Can you work these out from the model? Positions are in its coordinate system, mm. A direction names the side the tool comes from. Give positions to 0.01 mm unless a question says otherwise; leave off trailing zeros. Loops run counter-clockwise (first coordinate to the right, second up) from the corner with the lowest first, then second, coordinate; pieces in that order, holes last. Notation, with made-up numbers: M -39,-36.75 L 0,-36.75 A26 ccw 0,-8.75 Z; hole C 4,6.5 d2. An arc over 180 degrees is marked long. One line per item, written item: value. Start each with the question number.
from build123d import *

# Parameters (mm, degrees)
SKETCH2_R          = 27.5
CUT_EXTRUDE1_DEPTH = 4
CUT_EXTRUDE2_DEPTH = 28


with BuildPart() as part:
    # Sketch1 → Revolve1 (revolve)
    with BuildSketch(Plane(origin=(0, 0, 0), x_dir=(0, 0, -1), z_dir=(1, 0, 0))):
        with BuildLine():
            Line((0, 0), (43, 0))
            Line((43, 0), (43, -5))
            Line((43, -5), (44, -5))
            ThreePointArc((44, -5), (44.707106781, -4.707106781), (45, -4))
            Line((45, -4), (45, -1))
            ThreePointArc((45, -1), (44.121320344, 1.121320344), (42, 2))
            Line((42, 2), (41, 2))
            ThreePointArc((41, 2), (38.878679656, 2.878679656), (38, 5))
            Line((38, 5), (38, 9))
            ThreePointArc((38, 9), (37.121320344, 11.121320344), (35, 12))
            Line((35, 12), (0, 12))
            Line((0, 12), (0, 0))
        make_face()
    revolve(axis=Axis((0, 12, 0), (0, -1, 0)))

    # Sketch2 → Cut-Extrude1 (cut)
    with BuildSketch(Plane(origin=(0, 12, 0), x_dir=(1, 0, 0), z_dir=(0, 1, 0))):
        with Locations((0, -2.368290616)):
            Circle(SKETCH2_R)
    extrude(amount=-CUT_EXTRUDE1_DEPTH, mode=Mode.SUBTRACT)

    # Sketch3 → Cut-Extrude2 (cut)
    with BuildSketch(Plane(origin=(0, 12, 0), x_dir=(1, 0, 0), z_dir=(0, 1, 0))):
        with BuildLine():
            Line((-6.5, 32.565854692), (6.5, 32.565854692))
            ThreePointArc((6.5, 32.565854692), (9, 30.065854692), (6.5, 27.565854692))
            Line((6.5, 27.565854692), (-6.5, 27.565854692))
            ThreePointArc((-6.5, 27.565854692), (-9, 30.065854692), (-6.5, 32.565854692))
        make_face()
    extrude(amount=-CUT_EXTRUDE2_DEPTH, mode=Mode.SUBTRACT)


solid = part.part
Q1. If we section it at D-D, the plane y = 3.75: Write out the boundary of the cut face in (x, z), plus the area to 3 significant figures.
Q2. Which directions (+Z, -Z, +X, -X, +Y, -Y) give clear straight access to the entire face, cutting with the end or side of a thin tool? Please do faces 1 (the face through (0, 8, 2)), 2 (the face through (-42, -5, 10)), 3 (the face through (1, 0, -1)), 4 (the face through (-9, 6, -30)).
Q3. I need wall thicknesses on line 1 along X through (y, z) = (-3.15, 0); line 2 along Z through (x, y) = (37, -1.75); line 3 along Y through (x, z) = (11.5, -22). Which ranges of each line are inside material? Lowest first, please.
Q4. For P1, Ø1, axis at x = 18.5, y = 1.5, coming from the +Z side; P2, Ø8, axis at x = -1.5, y = 7, coming from the -Z side; P3, Ø10, axis at x = 13, z = 29.5, coming from the -Y side, each with a flat end and sliding along its axis, tell me the tip position at first contact or that it passes through.
Q5. If we section it at A-A, the plane x = 0: Write out the boundary of the cut face in (y, z), plus the area to 3 significant figures.
Q6. If we section it at C-C, the plane z = 0: Write out the boundary of the cut face in (x, y).
Q7. If we section it at B-B, the plane y = 10.75: Write out the boundary of the cut face in (x, z), plus the area to 3 significant figures.
Response:
1. outline: C 0,0 d76.55; hole M -6.5,-32.57 L 6.5,-32.57 A2.5 ccw 6.5,-27.57 L -6.5,-27.57 A2.5 ccw Z
1. area: 4,520 mm^2
2. face 1: +Y
2. face 2: +Z, -Z, +X, -X, -Y
2. face 3: -Y
2. face 4: +Y, -Y
3. line 1: -45 to -43, 43 to 45
3. line 2: -25.61 to -21.91, 21.91 to 25.61
3. line 3: 0 to 8
4. P1: z = 40.23
4. P2: z = -38.74
4. P3: y = 0
5. outline: M -5,-44 A1 ccw -4,-45 L -1,-45 A3 ccw 2,-42 L 2,-41 A3 cw 5,-38 L 9,-38 A3 ccw 12,-35 L 12,-32.57 L 0,-32.57 L 0,-43 L -5,-43 Z; M -5,43 L 0,43 L 0,-27.57 L 12,-27.57 L 12,-25.13 L 8,-25.13 L 8,29.87 L 12,29.87 L 12,35 A3 ccw 9,38 L 5,38 A3 cw 2,41 L 2,42 A3 ccw -1,45 L -4,45 A1 ccw -5,44 Z
5. area: 676 mm^2
6. outline: M -45,-4 A1 ccw -44,-5 L -43,-5 L -43,0 L 43,0 L 43,-5 L 44,-5 A1 ccw 45,-4 L 45,-1 A3 ccw 42,2 L 41,2 A3 cw 38,5 L 38,9 A3 ccw 35,12 L 27.4,12 L 27.4,8 L -27.4,8 L -27.4,12 L -35,12 A3 ccw -38,9 L -38,5 A3 cw -41,2 L -42,2 A3 ccw -45,-1 Z
7. outline: C 0,0 d74.87; hole C 0,2.37 d55; hole M -6.5,-32.57 L 6.5,-32.57 A2.5 ccw 6.5,-27.57 L -6.5,-27.57 A2.5 ccw Z
7. area: 1,940 mm^2
